Source: three-view drawing plus pictorial views. Frame: mm from the lowest corner of the part. Give positions to 0.01 mm unless a question says otherwise; leave off trailing zeros. Write each loop counter-clockwise with the first axis right and the second up, starting at its lowest first coordinate (ties: lowest second). Pieces come first, ordered by that corner, then holes.
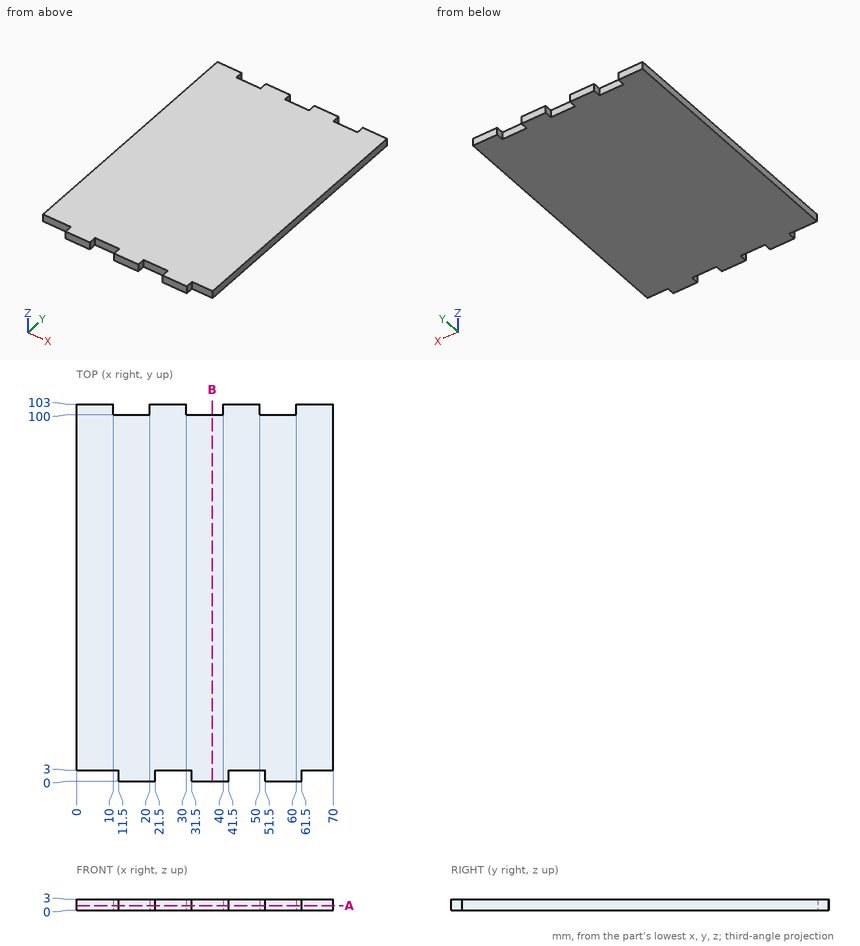
Q1. Section B-B on x = 37. Output: boundary loops of the cut face in (y, z), plus the area to 3 significant figures.
Filled sheet:
outline: (0, 0) - (100, 0) - (100, 3) - (0, 3) - close
area: 300 mm2
Q2. Section A-A on z = 1.3. Output: boundary loops of the cut face in (x, y), plus the area to 3 significant figures.
Filled sheet:
outline: (0, 3) - (11.5, 3) - (11.5, 0) - (21.5, 0) - (21.5, 3) - (31.5, 3) - (31.5, 0) - (41.5, 0) - (41.5, 3) - (51.5, 3) - (51.5, 0) - (61.5, 0) - (61.5, 3) - (70, 3) - (70, 103) - (60, 103) - (60, 100) - (50, 100) - (50, 103) - (40, 103) - (40, 100) - (30, 100) - (30, 103) - (20, 103) - (20, 100) - (10, 100) - (10, 103) - (0, 103) - close
area: 7,000 mm2
Q3. Ray query, line 1 along Y through (x, z) = (44.5, 0.8); line 2 along Y through (x, z) = (15.5, 0.9). Return the intervals inside material, ascending.
Filled sheet:
line 1: y = 3 to 103
line 2: y = 0 to 100
Q4. Pin query (flat end, axial travel): P1, Ø1, axis at x = 30.5, z = 1.5, coming from the -Y side; P2, Ø0.9, axis at y = 1.5, z = 1.5, coming from the +X side; P3, Ø0.9, axis at y = 1.5, z = 1.5, coming from the -X side. Return the tip coordinate at first contact, or that it passes through.
Filled sheet:
P1: stops at y = 3
P2: stops at x = 61.5
P3: stops at x = 11.5
